from build123d import *

# Parameters (mm, degrees)
F1_DEPTH = 15
F2_R     = 2
F3_DEPTH = 25


with BuildPart() as f1:
    # F0 (on Top) → F1 (new body)
    with BuildSketch(Plane.XY):
        with BuildLine():
            ThreePointArc((10, 7), (0, 17), (-10, 7))
            Line((-10, 7), (-10, 5))
            Line((-10, 5), (-20, 5))
            Line((-20, 5), (-20, 0))
            Line((-20, 0), (-6, 0))
            Line((-6, 0), (-6, 6))
            ThreePointArc((-6, 6), (0, 12), (6, 6))
            Line((6, 6), (6, 0))
            Line((6, 0), (20, 0))
            Line((20, 0), (20, 5))
            Line((20, 5), (10, 5))
            Line((10, 5), (10, 7))
        make_face()
    extrude(amount=F1_DEPTH)

    # F2 (on Front) → F3 (cut)
    with BuildSketch(Plane.XZ):
        with Locations((-14.142513, 7.235705)):
            Circle(F2_R)
        with Locations((14.142513, 7.235705)):
            Circle(F2_R)
    extrude(amount=-F3_DEPTH, mode=Mode.SUBTRACT)


solid = f1.part
Can you work these out from the model? Positions are in its coordinate system, mm. A direction names the side the tool comes from. Give positions to 0.01 mm unless a question says otherwise; leave off trailing zeros. Write each loop counter-clockwise with the first axis right and the second up, starting at its lowest first coordinate (ties: lowest second). Pieces come first, ordered by that corner, then holes. Notation, with made-up numbers: M 80,30 L 113,30 A12 cw 113,35 Z; hole C -37.75,18.5 d6. An arc over 180 degrees is marked long. Answer in a Markdown table with one row per item. Add a question column.
Item 1: Please list where these lines run through material, in increasing order: L1, parallel to X at y = 4.5, z = 7.25; L2, parallel to X at y = 3.25, z = 8.25; L3, parallel to X at y = 3, z = 3.25.
Item 2: On a 3-axis mill with a long thin cutter (end or side, diameter ignored), from which of +Z, -Z, +X, -X, +Y, -Y can I reach the whole of each face in a straight line? I mean faces 1 (the flat face through (-16, 5, 9)), 2 (the flat face through (6, 3, 7)), 3 (the flat face through (10, 6, 7)). Say none if no direction works.
Item 3: Imagine slicing it at B-B, the plane z = 13.75. Write out the boundary of the cut face in (x, y).
Item 4: Imagine slicing it at D-D, the plane z = 6.75. Write out the boundary of the cut face in (x, y), plus the area to 3 significant figures.
Item 5: Imagine slicing it at A-A, the plane y = 3.5. Write out the boundary of the cut face in (x, z), plus the area to 3 significant figures.
Item 6: Imagine slicing it at C-C, the plane y = 9. Write out the boundary of the cut face in (x, z).
Item 7: For pin 1 Ø1.5 at (x, y) = (5, 2.5) entering from +Z; pin 2 Ø2 at (y, z) = (9.5, 3) entering from -X; pin 3 Ø5 at (x, z) = (14.14, 7.24) entering from +Y; pin 4 Ø1 at (y, z) = (6.5, 5.5) entering from +X, each with a flat end and sliding along its axis, tell me the tip position at first contact or that it passes through.
Item 8: We'd pull the mould along X, two halves only. Please class faces 4 (the flat face through (-10, 6, 7)), 5 (the cylindrical face through (0, 17, 7)), 6 (the flat face through (16, 5, 9)), 7 (the flat face through (-6, 3, 7)): released by +X, released by -X, zero draft, split by the parting line, or undercut.
Evaluation:
| question | item | result |
|---|---|---|
| 1 | L1 | x = -20 to -16.14, -12.14 to -6, 6 to 12.14, 16.14 to 20 |
| 1 | L2 | x = -20 to -15.87, -12.42 to -6, 6 to 12.42, 15.87 to 20 |
| 1 | L3 | x = -20 to -6, 6 to 20 |
| 2 | face 1 | +Z, -Z, -X, +Y |
| 2 | face 2 | +Z, -Z, -Y |
| 2 | face 3 | +Z, -Z, +X, +Y |
| 3 | outline | M -20,0 L -6,0 L -6,6 A6 cw 6,6 L 6,0 L 20,0 L 20,5 L 10,5 L 10,7 A10 ccw -10,7 L -10,5 L -20,5 Z |
| 4 | outline | M -20,0 L -16.08,0 L -16.08,5 L -20,5 Z; M -12.2,0 L -6,0 L -6,6 A6 cw 6,6 L 6,0 L 12.2,0 L 12.2,5 L 10,5 L 10,7 A10 ccw -10,7 L -10,5 L -12.2,5 Z; M 16.08,0 L 20,0 L 20,5 L 16.08,5 Z |
| 4 | area | 230 mm² |
| 5 | outline | M -20,0 L -6,0 L -6,15 L -20,15 Z; M 6,0 L 20,0 L 20,15 L 6,15 Z; hole C -14.14,7.24 d4; hole C 14.14,7.24 d4 |
| 5 | area | 395 mm² |
| 6 | outline | M -9.8,0 L -5.2,0 L -5.2,15 L -9.8,15 Z; M 5.2,0 L 9.8,0 L 9.8,15 L 5.2,15 Z |
| 7 | pin 1 | passes through |
| 7 | pin 2 | stops at x = -9.89 |
| 7 | pin 3 | stops at y = 5 |
| 7 | pin 4 | stops at x = 10 |
| 8 | face 4 | released by -X |
| 8 | face 5 | split by the parting line |
| 8 | face 6 | zero draft |
| 8 | face 7 | undercut |
